Can you work these out from the model? Positions are in its coordinate system, mm. Coordinates: 2 decimals unless noted, no trailing zeros. Loops run counter-clockwise (first coordinate to the right, second up) from the corner with the lowest first, then second, coordinate; pieces in that order, holes last. Notation, with made-up numbers: (-19.75, 27.25) -> (24.25, 27.25) arc R23 ccw to (24.25, 57.25) -> close; hole circle Ø9 at (21.25, 63). An arc over 180 degrees is marked (long way). Put each result on its own line as item: value. Start each with the question number.
Item 1: If we section it at D-D on x = -39: Please give me the cut outline in (y, z).
Item 2: Will this pin go through, and if not, where does the flat tip stop? P1, Ø3, axis at x = -6.6, y = 17.5, coming from the +Z side.
Item 3: Please list where these lines run through material, in increasing order: L1, parallel to Y at x = -6.6, z = 1.45; L2, parallel to X at y = 17, z = 1.9; L3, parallel to X at y = -19, z = 1.1. Write a range as from..to.
Item 4: If we section it at B-B on x = 6.6: Please give me the cut outline in (y, z).
Item 5: If we section it at A-A on y = 17.5: Please give me the cut outline in (x, z).
Item 6: If we section it at C-C on z = 0.3: State how many separate pieces and enclosed holes the cut face has, plus the area to 3 significant figures.
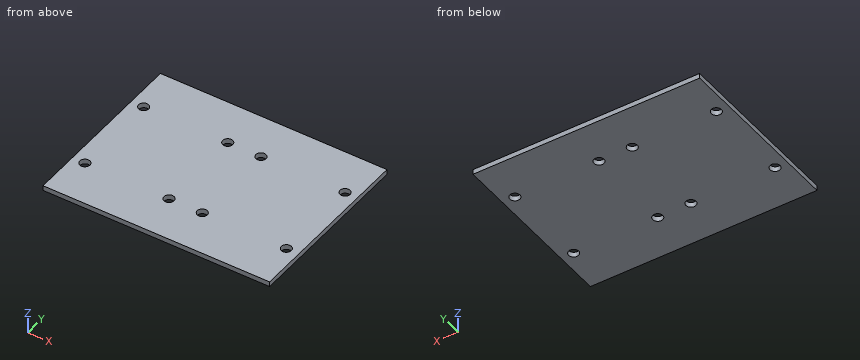
```python
from build123d import *

# Parameters (mm, degrees)
SKETCH1_W           = 90
SKETCH1_H           = 70
SKETCH1_R           = 2
BOSS_EXTRUDE1_DEPTH = 2


with BuildPart() as part:
    # Sketch1 → Boss-Extrude1 (new body)
    with BuildSketch(Plane.XY):
        Rectangle(SKETCH1_W, SKETCH1_H)
        with Locations((-6.6, 17.5)):
            Circle(SKETCH1_R, mode=Mode.SUBTRACT)
        with Locations((6.6, 17.5)):
            Circle(SKETCH1_R, mode=Mode.SUBTRACT)
        with Locations((-6.6, -17.5)):
            Circle(SKETCH1_R, mode=Mode.SUBTRACT)
        with Locations((-40, 17.5)):
            Circle(SKETCH1_R, mode=Mode.SUBTRACT)
        with Locations((-40, -17.5)):
            Circle(SKETCH1_R, mode=Mode.SUBTRACT)
        with Locations((40, 17.5)):
            Circle(SKETCH1_R, mode=Mode.SUBTRACT)
        with Locations((6.6, -17.5)):
            Circle(SKETCH1_R, mode=Mode.SUBTRACT)
        with Locations((40, -17.5)):
            Circle(SKETCH1_R, mode=Mode.SUBTRACT)
    extrude(amount=BOSS_EXTRUDE1_DEPTH)


solid = part.part
```
Solutions:
1. outline: (-35, 0) -> (-19.23, 0) -> (-19.23, 2) -> (-35, 2) -> close; (-15.77, 0) -> (15.77, 0) -> (15.77, 2) -> (-15.77, 2) -> close; (19.23, 0) -> (35, 0) -> (35, 2) -> (19.23, 2) -> close
2. P1: through
3. L1: -35..-19.5, -15.5..15.5, 19.5..35
3. L2: -45..-41.94, -38.06..-8.54, -4.66..4.66, 8.54..38.06, 41.94..45
3. L3: -45..-41.32, -38.68..-7.92, -5.28..5.28, 7.92..38.68, 41.32..45
4. outline: (-35, 0) -> (-19.5, 0) -> (-19.5, 2) -> (-35, 2) -> close; (-15.5, 0) -> (15.5, 0) -> (15.5, 2) -> (-15.5, 2) -> close; (19.5, 0) -> (35, 0) -> (35, 2) -> (19.5, 2) -> close
5. outline: (-45, 0) -> (-42, 0) -> (-42, 2) -> (-45, 2) -> close; (-38, 0) -> (-8.6, 0) -> (-8.6, 2) -> (-38, 2) -> close; (-4.6, 0) -> (4.6, 0) -> (4.6, 2) -> (-4.6, 2) -> close; (8.6, 0) -> (38, 0) -> (38, 2) -> (8.6, 2) -> close; (42, 0) -> (45, 0) -> (45, 2) -> (42, 2) -> close
6. separate pieces: 1
6. enclosed holes: 8
6. area: 6,200 mm^2
